Work out the finished part from the listing and answer in its coordinate system (mm). Face numbers are marked on the shaded views. A direction names the side the tool comes from. Give positions to 0.01 mm unless a question says otherwise; leave off trailing zeros. Write each loop counter-clockwise with the first axis right and the second up, starting at its lowest first coordinate (ties: lowest second). Pieces come first, ordered by that corner, then holes. Notation, with made-up numbers: (89, 33.25) - (125, 33.25) arc R28 cw to (125, 56.25) - close; hole circle Ø9 at (-14.75, -26). An arc over 180 degrees is marked (long way). Write item = value, one per line.
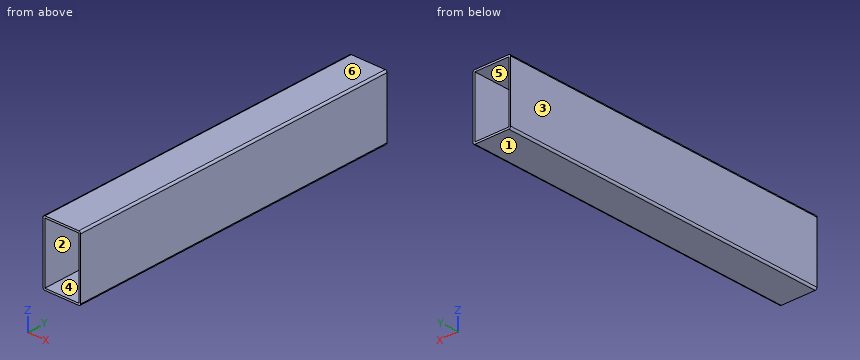
Autodesk Inventor part; units mm, degrees
ref_plane "YZ Plane" through (0, 0, 0) normal (1, 0, 0) x (0, 1, 0)
ref_plane "XZ Plane" through (0, 0, 0) normal (0, 1, 0) x (-1, 0, 0)
ref_plane "XY Plane" through (0, 0, 0) normal (0, 0, 1) x (1, 0, 0)
sketch "Sketch1" plane through (0, 0, 0) normal (0, 1, 0) x (-1, 0, 0)
  line L0 (30, -50) -> (-30, -50)
  line L1 (-30, -50) -> (-30, 50)
  line L2 (-30, 50) -> (30, 50)
  line L3 (30, 50) -> (30, -50)
  line L4 (30, -50) -> (-30, 50) construction
  line L5 (-30, -50) -> (30, 50) construction
  point P0 (0, 0)
  dimension "d0" = 60
  dimension "d1" = 100
extrude "Extrusion1" add sketch "Sketch1" along normal mid plane 532.5
fillet "Fillet1" radius 3 4 edges at (-30, 0, 50) (30, 0, 50) (30, 0, -50) (-30, 0, -50)
shell "Shell1" thickness 3 removed faces 2 at (10, -266.25, 15.6667) at (10, 266.25, 15.6667)
properties part number "Perfil refuerzo"
1. Find section A-A, the plane z = 6.5. Give the vertices of the cut face in (x, y).
Solution:
outline = (-30, -266.25) - (-27, -266.25) - (-27, 266.25) - (-30, 266.25) - close; (27, -266.25) - (30, -266.25) - (30, 266.25) - (27, 266.25) - close
2. Given pin 1 (5 mm diameter, centred on x = -23.5, z = 37, fed in from -Y), flat-ended and moving along its own axis, determine where the tip first touches the part or whether it passes through.
Solution:
pin_1 = through
3. A tool of negligible diameter and unlimited length cuts with its end or side. For the marked faces 1 and 2, from which of +Z, -Z, +X, -X, +Y, -Y can it reach the whole face along a straight path? Write none if from no direction.
Solution:
face_1 = -Z, +X, -X, +Y, -Y
face_2 = +Y, -Y
4. Straight lines are drawn through the part: line 1 (X direction, y = 59.5, z = -39); line 2 (Z direction, x = -4, y = -241.5); line 3 (Z direction, x = 28, y = -2). For each, find the intervals that lie inside material, in ascending order.
Solution:
line_1 = -30 to -27, 27 to 30
line_2 = -50 to -47, 47 to 50
line_3 = -49.83 to 49.83
5. For a pull along Z with two mould halves and no side action, classify the marked faces 3, 4, 5 and 6 as pulls with the +Z half, pulls with the -Z half, needs draft (parallel to the pull), parting line crosses it, or undercut.
Solution:
face_3 = needs draft
face_4 = undercut
face_5 = undercut
face_6 = pulls with the +Z half
6. Find section C-C, the plane x = -4. Give the vertices of the cut face in (y, z), then the cut area to 4 significant figures.
Solution:
outline = (-266.25, -50) - (266.25, -50) - (266.25, -47) - (-266.25, -47) - close; (-266.25, 47) - (266.25, 47) - (266.25, 50) - (-266.25, 50) - close
area = 3,195 mm^2
7. Find section B-B, the plane y = 64. Give the vertices of the cut face in (x, z), then the cut area to 3 significant figures.
Solution:
outline = (-30, -47) arc R3 ccw to (-27, -50) - (27, -50) arc R3 ccw to (30, -47) - (30, 47) arc R3 ccw to (27, 50) - (-27, 50) arc R3 ccw to (-30, 47) - close; hole (-27, -47) - (27, -47) - (27, 47) - (-27, 47) - close
area = 916 mm^2
